The listing builds one solid part. Answer for the finished solid, in the listing's coordinates (mm). A direction names the side the tool comes from. Round coordinates to 2 decimals unless told otherwise and drop trailing zeros. Write each loop counter-clockwise with the first axis right and the second up, starting at its lowest first coordinate (ties: lowest second). Pieces come first, ordered by that corner, then holes. Notation, with made-up numbers: (44.25, 28) - (70.25, 28) arc R26 ccw to (70.25, 47) - close; hole circle Ø5 at (-39, -27.75). An arc over 180 degrees is marked (long way). Answer in a Markdown table with one row per item.
from build123d import *

# Parameters (mm, degrees)
BOSS_EXTRUDE1_START = -8.805333
SKETCH5_R           = 17.197916667
BOSS_EXTRUDE1_DEPTH = 13.208
SKETCH6_R           = 16.09725
CUT_EXTRUDE1_DEPTH  = 14.675555556


# Read off the part's stored shape, not the designer's step: LPattern1
with BuildPart() as part:
    # Sketch4 → Revolve2 (revolve)
    with BuildSketch(Plane.XY, mode=Mode.PRIVATE) as revolve2_sk:
        with BuildLine():
            Line((0, 8.805333333), (0, 4.402666667))
            Line((0, 4.402666667), (21.05025, 4.402666667))
            ThreePointArc((21.05025, 4.402666667), (19.760738789, 7.515822122), (16.647583333, 8.805333333))
            Line((16.647583333, 8.805333333), (0, 8.805333333))
        make_face()
        Polygon((0, 2.685626667), (19.536840212, 2.685626667), (19.536840212, 2.157306667), (17.197916667, 0.572346667), (0, 0.572346667), align=None)
    revolve(revolve2_sk.sketch.rotate(Axis((0, -8.805333333, 0), (0, 1, 0)), 90), axis=Axis((0, -8.805333333, 0), (0, 1, 0)))



with BuildPart() as body_2:
    # LPattern1 outline → LPattern1 (revolve)
    with BuildSketch(Plane.XY):
        Polygon((19.536840212, -5.503333333), (19.536840212, -4.975013333), (0, -4.975013333), (0, -7.088293333), (17.197916667, -7.088293333), align=None)
        Polygon((0, -1.144693333), (0, -3.257973333), (17.197916667, -3.257973333), (19.536840213, -1.673013333), (19.536840212, -1.144693333), align=None)
    revolve(axis=Axis((0, 0, 0), (0, 1, 0)))


with BuildPart() as part_1:
    add(part.part)

    add(body_2.part)  # Boss-Extrude1 merges body 2
    # Sketch5 → Boss-Extrude1 (add)
    with BuildSketch(Plane(origin=(0, 0, 0), x_dir=(1, 0, 0), z_dir=(0, 1, 0)).offset(BOSS_EXTRUDE1_START)):
        with Locations(Location((0, 0, 0), (0, 0, 90))):
            Circle(SKETCH5_R)
    extrude(amount=BOSS_EXTRUDE1_DEPTH)

    # Sketch6 → Cut-Extrude1 (cut)
    with BuildSketch(Plane.XZ.offset(8.805333333)):
        with Locations(Location((0, 0, 0), (0, 0, 270))):
            Circle(SKETCH6_R)
    extrude(amount=-CUT_EXTRUDE1_DEPTH, mode=Mode.SUBTRACT)


solid = part_1.part
(1) Flat-ended cylindrical pins translate along their axes: pin 1 (6 mm diameter, centred on y = -6.5, z = 9.5, fed in from +X); pin 2 (12.5 mm diameter, centred on x = -9, z = 0, fed in from -Y); pin 3 (2 mm diameter, centred on y = 1.5, z = 4, fed in from +X). Find the tip coordinate at first contact, or state that the pin passes through.
Checked values:
| item | result |
|---|---|
| pin 1 | stops at x = 18.36 |
| pin 2 | stops at y = 5.87 |
| pin 3 | stops at x = 19.27 |
(2) For a pull along Z with two mould halves and no side action, classify faces 4 (the flat face through (1.4, -4.975, 17.3)), 5 (the cylindrical face through (15.96, -1.57, 2.1)), 6 (the cylindrical face through (-5.868, 2.418, -18.635)) as pulls with the +Z half, pulls with the -Z half, needs draft (parallel to the pull), parting line crosses it, or undercut.
Checked values:
| item | result |
|---|---|
| face 4 | needs draft |
| face 5 | undercut |
| face 6 | parting line crosses it |
(3) Section A-A (y = 3.5) is taken. Give the vertices of the cut face in (x, z).
Checked values:
| item | result |
|---|---|
| outline | circle Ø34.4 at (0, 0); hole circle Ø32.19 at (0, 0) |
(4) For faces 1 (the flat face through (0, 8.805, 0)), 2 (the cylindrical face through (18.635, -5.235, -5.868)), 3 (the flat face through (1.4, -1.145, 17.3)), determine the directions among +Z, -Z, +X, -X, +Y, -Y from which every point of the face is accessible in a straight line to the end or side of a thin tool.
Checked values:
| item | result |
|---|---|
| face 1 | +Z, -Z, +X, -X, +Y |
| face 2 | -Y |
| face 3 | none |
(5) Find the intervals of material crossed by line 1 (Y direction, x = -3.5, z = -17); line 2 (X direction, y = -0.5, z = -0.5); line 3 (X direction, y = -5.25, z = 0), in increasing order.
Checked values:
| item | result |
|---|---|
| line 1 | y = -6.98 to -4.98, -3.15 to -1.14, 0.68 to 2.69, 4.4 to 8.75 |
| line 2 | x = -17.19 to -16.09, 16.09 to 17.19 |
| line 3 | x = -19.54 to -16.1, 16.1 to 19.54 |
(6) Section B-B (y = 1.25) is taken. Give the vertices of the cut face in (x, z).
Checked values:
| item | result |
|---|---|
| outline | circle Ø36.4 at (0, 0); hole circle Ø32.19 at (0, 0) |
